The drawing under review shows one solid part. Ordinate dimensions are in mm from its lowest x, y, z. Give positions to 0.01 mm unless a question says otherwise; leave off trailing zeros. Order: outer loops, then holes, each group sorted by start corner. A loop starts at its lowest first (then second) coordinate and runs counter-clockwise, first axis right, second up. Notation, with made-up numbers: (-25.75, 74) - (-8.75, 74) arc R3 ccw to (-8.75, 78) - close; hole circle Ø7 at (16, 53.25). An arc over 180 degrees is marked (long way). Write item = value, one per line. Start each with the question number.
1. Wall thickness on probe 1 along Y at (x, z) = (190, 12.25); probe 2 along X at (y, z) = (212, 18); probe 3 along X at (y, z) = (113, 13.5) (1 decimal): over which ranges is each line inside the solid? List them lowest first.
2. We need section B-B, the plane x = 190. Give the boundary of the cut face in (y, z).
3. We need section C-C, the plane y = 40. Give the boundary of the cut face in (x, z).
4. We need section D-D, the plane z = 9. State how many separate pieces and enclosed holes the cut face has, and give its area (3 significant figures).
5. For P1, Ø11, axis at y = 140.5, z = 11.5, coming from the +X side; P2, Ø8, axis at y = 32, z = 12, coming from the +X side; P3, Ø4, axis at x = 134.5, y = 197, coming from the -Z side; P4, Ø2, axis at x = 87.5, y = 96, coming from the -Z side, all flat-tipped, find the tip position at first contact; note any pin that passes through.
6. Mouldability with a two-part tool opening along X and no side actions: class the marked faces 1 and 2 as pulls with the +X half, pulls with the -X half, needs draft (parallel to the pull), parting line crosses it, or undercut.
7. We need section A-A, the plane y = 126.6. Give the boundary of the cut face in (x, z), and give its area (3 significant figures).
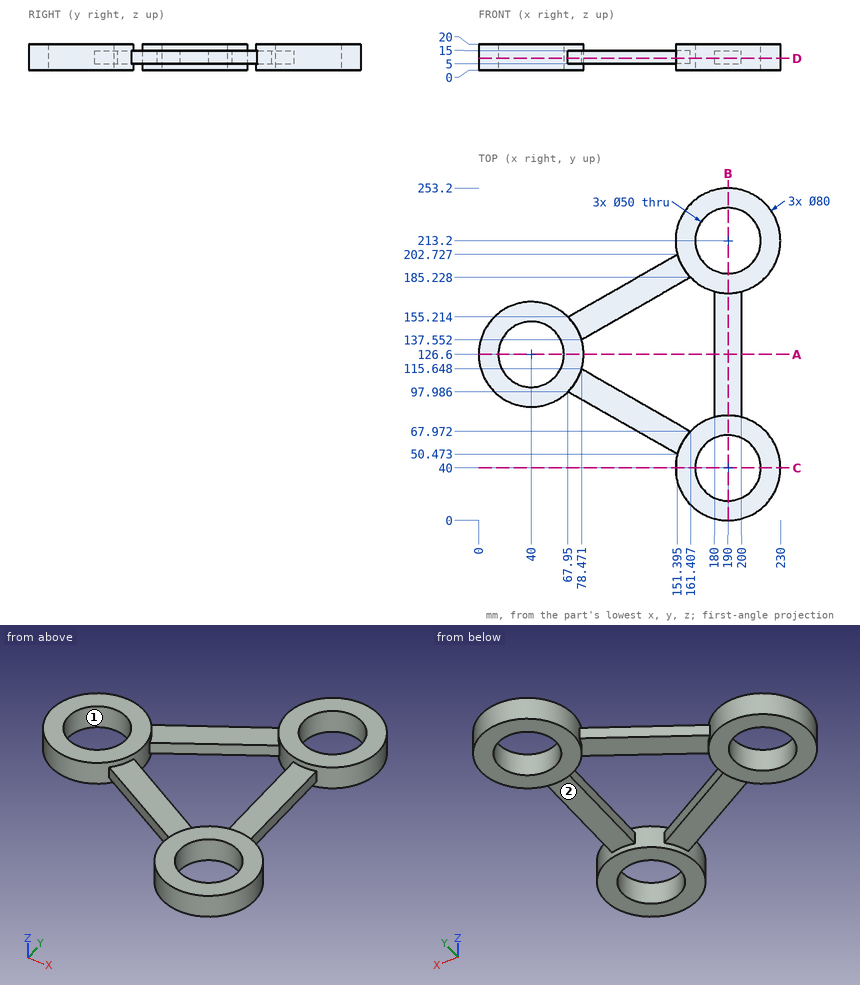
Model answer:
q1.probe_1 = 0 to 15, 65 to 188.2, 238.2 to 253.2
q1.probe_2 = 150.02 to 165.03, 214.97 to 229.98
q1.probe_3 = 2.4 to 19, 61 to 83.1, 180 to 200
q2.outline = (0, 0) - (15, 0) - (15, 20) - (0, 20) - close; (65, 0) - (80, 0) - (80, 5) - (173.2, 5) - (173.2, 0) - (188.2, 0) - (188.2, 20) - (173.2, 20) - (173.2, 15) - (80, 15) - (80, 20) - (65, 20) - close; (238.2, 0) - (253.2, 0) - (253.2, 20) - (238.2, 20) - close
q3.outline = (150, 0) - (165, 0) - (165, 20) - (150, 20) - close; (215, 0) - (230, 0) - (230, 20) - (215, 20) - close
q4.separate_pieces = 1
q4.enclosed_holes = 4
q4.area = 14,900 mm2
q5.P1 = 200
q5.P2 = 229.8
q5.P3 = through
q5.P4 = 5
q6.face_1 = undercut
q6.face_2 = needs draft
q7.outline = (0, 0) - (15, 0) - (15, 20) - (0, 20) - close; (65, 0) - (80, 0) - (80, 20) - (65, 20) - close; (180, 5) - (200, 5) - (200, 15) - (180, 15) - close
q7.area = 800 mm2
